```python
from build123d import *

# Parameters (mm, degrees)
BOSS_EXTRUDE1_DEPTH      = 9.5
BOSS_EXTRUDE1_DEPTH_BACK = 9.5
BOSS_EXTRUDE2_DEPTH      = 19
SKETCH4_R                = 1.45
CUT_EXTRUDE1_DEPTH       = 10
SKETCH5_R                = 1.5
CUT_EXTRUDE2_DEPTH       = 10
SKETCH6_R                = 1.45
CUT_EXTRUDE3_DEPTH       = 10
SKETCH7_R                = 1.45
CUT_EXTRUDE4_DEPTH       = 10


with BuildPart() as part:
    # Sketch2 → Boss-Extrude1 (new, two sides: drawn at the far end of the back side and taken through both)
    with BuildSketch(Plane(origin=(0, 0, 0), x_dir=(-1, 0, 0), z_dir=(0, 1, 0)).offset(-BOSS_EXTRUDE1_DEPTH_BACK)):
        Polygon((-23.95, 28.875), (-3.75, 28.875), (-3.75, -36.125), (3.75, -36.125), (3.75, 28.875), (23.95, 28.875), (23.95, -36.125), (31.45, -36.125), (31.45, 28.875), (51.65, 28.875), (51.65, -36.125), (56.65, -36.125), (56.65, 36.125), (-56.65, 36.125), (-56.65, -36.125), (-51.65, -36.125), (-51.65, 28.875), (-31.45, 28.875), (-31.45, -36.125), (-23.95, -36.125), align=None)
    extrude(amount=BOSS_EXTRUDE1_DEPTH + BOSS_EXTRUDE1_DEPTH_BACK)

    # Sketch3 → Boss-Extrude2 (add)
    with BuildSketch(Plane.XY.offset(36.125)):
        Polygon((-56.65, 9.5), (-62.25, 15.1), (-102.45, 15.1), (-102.45, 10.1), (-62.25, 10.1), (-62.25, -10.1), (-102.45, -10.1), (-102.45, -15.1), (-62.25, -15.1), (-56.65, -9.5), align=None)
    extrude(amount=-BOSS_EXTRUDE2_DEPTH)

    # Sketch4 → Cut-Extrude1 (cut)
    with BuildSketch(Plane.XY.offset(36.125)):
        with Locations((-57.5, 5)):
            Circle(SKETCH4_R)
        with Locations((-57.5, -5)):
            Circle(SKETCH4_R)
    extrude(amount=-CUT_EXTRUDE1_DEPTH, mode=Mode.SUBTRACT)

    # Sketch5 → Cut-Extrude2 (cut)
    with BuildSketch(Plane(origin=(0, 9.5, 0), x_dir=(-1, 0, 0), z_dir=(0, 1, 0))):
        with Locations(Location((-46.55, 33.625, 0), (0, 0, 90))):
            Circle(SKETCH5_R)
        with Locations(Location((-36.55, 33.625, 0), (0, 0, 90))):
            Circle(SKETCH5_R)
        with Locations(Location((8.85, 33.625, 0), (0, 0, 90))):
            Circle(SKETCH5_R)
        with Locations(Location((18.85, 33.625, 0), (0, 0, 90))):
            Circle(SKETCH5_R)
    extrude(amount=-CUT_EXTRUDE2_DEPTH, mode=Mode.SUBTRACT)

    # Sketch6 → Cut-Extrude3 (cut)
    with BuildSketch(Plane.XZ.offset(9.5)):
        with Locations(Location((-46.55, 33.625, 0), (0, 0, 270))):
            Circle(SKETCH6_R)
        with Locations(Location((-36.55, 33.625, 0), (0, 0, 270))):
            Circle(SKETCH6_R)
        with Locations(Location((9.254566693, 33.625, 0), (0, 0, 270))):
            Circle(SKETCH6_R)
        with Locations(Location((19.254566693, 33.625, 0), (0, 0, 270))):
            Circle(SKETCH6_R)
    extrude(amount=-CUT_EXTRUDE3_DEPTH, mode=Mode.SUBTRACT)

    # Sketch7 → Cut-Extrude4 (cut)
    with BuildSketch(Plane(origin=(0, 0, -36.125), x_dir=(1, 0, 0), z_dir=(0, 0, -1))):
        with Locations(Location((-27.7, 0, 0), (0, 0, 180))):
            Circle(SKETCH7_R)
        with Locations(Location((27.7, 0, 0), (0, 0, 180))):
            Circle(SKETCH7_R)
    extrude(amount=-CUT_EXTRUDE4_DEPTH, mode=Mode.SUBTRACT)


solid = part.part
```
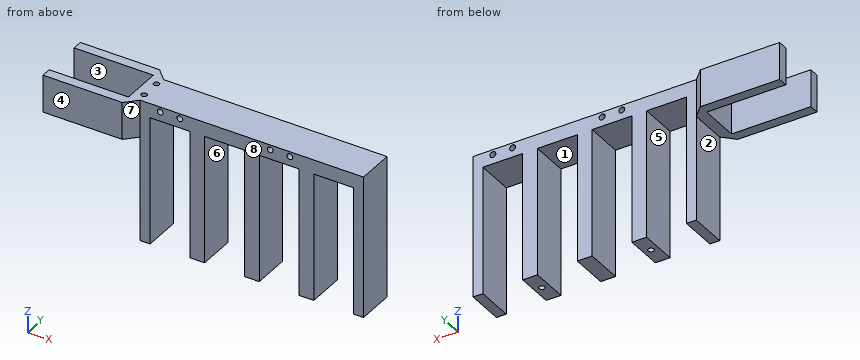
Could you check a few things on this model? Use its own coordinates, in mm. Face numbers are marked on the shaded views. A direction names the side the tool comes from. Coordinates: 2 decimals unless noted, no trailing zeros. Write each loop counter-clockwise with the first axis right and the second up, starting at its lowest first coordinate (ties: lowest second). Pieces come first, ordered by that corner, then holes. Notation, with made-up numbers: (55.25, -26) - (84.25, -26) arc R21 cw to (84.25, 10) - close; hole circle Ø11 at (16.25, -27). An arc over 180 degrees is marked (long way). Use a Markdown table: item, result.
Q1. Imagine slicing it at D-D (x = -36.55). List the corners of the cut face in (y, z) for me (3 decimals), and give its area (3 significant figures).
Geometry check:
| item | result |
|---|---|
| outline | (-9.5, 28.875) - (9.5, 28.875) - (9.5, 36.125) - (-9.5, 36.125) - (-9.5, 35.075) - (0.5, 35.075) - (0.5, 32.175) - (-9.5, 32.175) - close |
| area | 109 mm2 |
Q2. Imagine slicing it at B-B (z = 24). List the corners of the cut face in (x, y) for me, and give its area (3 significant figures).
Geometry check:
| item | result |
|---|---|
| outline | (-102.45, -15.1) - (-62.25, -15.1) - (-56.65, -9.5) - (-51.65, -9.5) - (-51.65, 9.5) - (-56.65, 9.5) - (-62.25, 15.1) - (-102.45, 15.1) - (-102.45, 10.1) - (-62.25, 10.1) - (-62.25, -10.1) - (-102.45, -10.1) - close; (-31.45, -9.5) - (-23.95, -9.5) - (-23.95, 9.5) - (-31.45, 9.5) - close; (-3.75, -9.5) - (3.75, -9.5) - (3.75, 9.5) - (-3.75, 9.5) - close; (23.95, -9.5) - (31.45, -9.5) - (31.45, 9.5) - (23.95, 9.5) - close; (51.65, -9.5) - (56.65, -9.5) - (56.65, 9.5) - (51.65, 9.5) - close |
| area | 1,160 mm2 |
Q3. I'm going to push flat-ended pins straight in: pin 1 Ø4 at (x, z) = (-18.85, 33.625) entering from -Y; pin 2 Ø15 at (x, y) = (-12.5, 2.5) entering from -Z (3 decimals); pin 3 Ø2.5 at (x, z) = (9.25, 33.62) entering from +Y. Where does each tip first touch, or does it pass through?
Geometry check:
| item | result |
|---|---|
| pin 1 | stops at y = -9.5 |
| pin 2 | stops at z = 28.875 |
| pin 3 | stops at y = 9.5 |
Q4. Imagine slicing it at A-A (z = -30). List the corners of the cut face in (x, y) for me.
Geometry check:
| item | result |
|---|---|
| outline | (-56.65, -9.5) - (-51.65, -9.5) - (-51.65, 9.5) - (-56.65, 9.5) - close; (-31.45, -9.5) - (-23.95, -9.5) - (-23.95, 9.5) - (-31.45, 9.5) - close; (-3.75, -9.5) - (3.75, -9.5) - (3.75, 9.5) - (-3.75, 9.5) - close; (23.95, -9.5) - (31.45, -9.5) - (31.45, 9.5) - (23.95, 9.5) - close; (51.65, -9.5) - (56.65, -9.5) - (56.65, 9.5) - (51.65, 9.5) - close; hole circle Ø2.9 at (-27.7, 0); hole circle Ø2.9 at (27.7, 0) |
Q5. Which directions (+Z, -Z, +X, -X, +Y, -Y) give clear straight access to the entire face, cutting with the end or side of a thin tool? Please do the marked faces 1, 2, 3 and 4.
Geometry check:
| item | result |
|---|---|
| face 1 | -Z, +Y, -Y |
| face 2 | -Z, -X, +Y, -Y |
| face 3 | +Z, -Z, -X |
| face 4 | +Z, -Z, +X, -X, -Y |
Q6. Please list where these lines run through material, in increasing order: L1, parallel to X at y = -4, z = -24; L2, parallel to X at y = 0, z = 25; L3, parallel to Y at x = -84.5, z = 31.
Geometry check:
| item | result |
|---|---|
| L1 | x = -56.65 to -51.65, -31.45 to -23.95, -3.75 to 3.75, 23.95 to 31.45, 51.65 to 56.65 |
| L2 | x = -62.25 to -51.65, -31.45 to -23.95, -3.75 to 3.75, 23.95 to 31.45, 51.65 to 56.65 |
| L3 | y = -15.1 to -10.1, 10.1 to 15.1 |
Q7. Thinking about a two-plate mould opening in X: for the marked faces 5, 6, 7 and 8, which applies, +X half, -X half, draft (parallel to the pull), parting line (faces both ways), or undercut?
Geometry check:
| item | result |
|---|---|
| face 5 | undercut |
| face 6 | undercut |
| face 7 | +X half |
| face 8 | draft |
Q8. Imagine slicing it at C-C (x = -78.5). List the corners of the cut face in (y, z) for me (3 decimals), and give its area (3 significant figures).
Geometry check:
| item | result |
|---|---|
| outline | (-15.1, 17.125) - (-10.1, 17.125) - (-10.1, 36.125) - (-15.1, 36.125) - close; (10.1, 17.125) - (15.1, 17.125) - (15.1, 36.125) - (10.1, 36.125) - close |
| area | 190 mm2 |
